Check sheet for the modelled part. Datum: model origin and axes. Units: mm. Face numbers are marked on the shaded views. A direction names the side the tool comes from. Coordinates: 2 decimals unless noted, no trailing zeros. Write each loop counter-clockwise with the first axis right and the second up, starting at its lowest first coordinate (ties: lowest second). Pieces come first, ordered by that corner, then holes. Notation, with made-up numbers: (12, 52) -> (51, 52) arc R6 ccw to (51, 60) -> close; hole circle Ø2 at (89, 63.5). An arc over 180 degrees is marked (long way). Put each result on its own line as item: value.
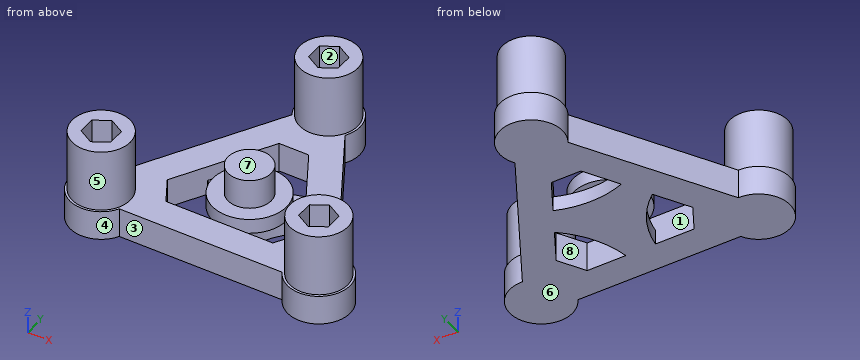
```python
from build123d import *

# Parameters (mm, degrees)
BOSS_EXTRUDE1_DEPTH = 5
BOSS_EXTRUDE2_DEPTH = 5
SKETCH4_R           = 9.75
BOSS_EXTRUDE3_DEPTH = 21
SKETCH5_R           = 12.441578391
BOSS_EXTRUDE4_DEPTH = 5
SKETCH5_3_R         = 7.25
BOSS_EXTRUDE5_DEPTH = 15
CHAMFER1_SIZE       = 10
CUT_EXTRUDE1_DEPTH  = 10


with BuildPart() as part:
    # Sketch2 → Boss-Extrude1 (new body, symmetric)
    with BuildSketch(Plane.XY):
        with BuildLine():
            ThreePointArc((8.946673347, 36.860907204), (0, 52.857), (-8.946673347, 36.860907204))
            Line((-8.946673347, 36.860907204), (-36.395818719, -10.682407204))
            ThreePointArc((-36.395818719, -10.682407204), (-45.775504768, -26.4285), (-27.449145372, -26.1785))
            Line((-27.449145372, -26.1785), (27.449145372, -26.1785))
            ThreePointArc((27.449145372, -26.1785), (45.775504768, -26.4285), (36.395818719, -10.682407204))
            Line((36.395818719, -10.682407204), (8.946673347, 36.860907204))
        make_face()
        Polygon((-28.02198399, -16.1785), (0, 32.357), (28.02198399, -16.1785), align=None, mode=Mode.SUBTRACT)
    extrude(amount=BOSS_EXTRUDE1_DEPTH, both=True)

    # Sketch3 → Boss-Extrude2 (add)
    with BuildSketch(Plane.XY):
        with BuildLine():
            Line((-16.510991995, 3.759122981), (-11.510991995, 12.419377019))
            ThreePointArc((-11.510991995, 12.419377019), (0, 10.282645658), (11.510991995, 12.419377019))
            Line((11.510991995, 12.419377019), (16.510991995, 3.759122981))
            ThreePointArc((16.510991995, 3.759122981), (8.905032358, -5.141322829), (5, -16.1785))
            Line((5, -16.1785), (-5, -16.1785))
            ThreePointArc((-5, -16.1785), (-8.905032358, -5.141322829), (-16.510991995, 3.759122981))
        make_face()
    extrude(amount=-BOSS_EXTRUDE2_DEPTH)

    # Sketch4 → Boss-Extrude3 (add)
    with BuildSketch(Plane.XY.offset(5)):
        with Locations((-36.682238028, -21.1785)):
            Circle(SKETCH4_R)
        with Locations((36.682238028, -21.1785)):
            Circle(SKETCH4_R)
        with Locations((0, 42.357)):
            Circle(SKETCH4_R)
    extrude(amount=BOSS_EXTRUDE3_DEPTH)

    # Sketch5 → Boss-Extrude4 (add)
    with BuildSketch(Plane.XY):
        Circle(SKETCH5_R)
    extrude(amount=BOSS_EXTRUDE4_DEPTH)

    # Sketch5<3> → Boss-Extrude5 (add)
    with BuildSketch(Plane.XY):
        Circle(SKETCH5_3_R)
    extrude(amount=BOSS_EXTRUDE5_DEPTH)

    # Chamfer1
    chamfer1_edges = [part.edges().sort_by_distance(p)[0] for p in [
        (28.02198399, -16.1785, 0),
        (-28.02198399, -16.1785, 0),
        (0, 32.357, 0),
    ]]
    chamfer(chamfer1_edges, length=CHAMFER1_SIZE)

    # Sketch8 → Cut-Extrude1 (cut)
    with BuildSketch(Plane.XY.offset(26)):
        Polygon((-41.682238028, -24.065251346), (-36.682238028, -26.952002692), (-31.682238028, -24.065251346), (-31.682238028, -18.291748654), (-36.682238028, -15.404997308), (-41.682238028, -18.291748654), align=None)
        Polygon((41.682238028, -24.065251346), (41.682238028, -18.291748654), (36.682238028, -15.404997308), (31.682238028, -18.291748654), (31.682238028, -24.065251346), (36.682238028, -26.952002692), align=None)
        Polygon((0, 48.130502692), (-5, 45.243751346), (-5, 39.470248654), (0, 36.583497308), (5, 39.470248654), (5, 45.243751346), align=None)
    extrude(amount=-CUT_EXTRUDE1_DEPTH, mode=Mode.SUBTRACT)


solid = part.part
```
Q1. Cross-section at B-B (z = 20). State how many separate pieces and enclosed holes the cut face has, plus the area to 3 significant figures.
Recorded:
separate pieces: 3
enclosed holes: 3
area: 636 mm2
Q2. Tool access check on the marked faces 5, 6, 7 and 8. Record the directions out of +Z, -Z, +X, -X, +Y, -Y that give a thin tool (end or side, any length) a straight path to the whole face; none if there is none.
Recorded:
face 5: +Z
face 6: -Z, +X, -X, +Y, -Y
face 7: +Z, +X, -X, -Y
face 8: +Z, -Z
Q3. Cross-section at A-A (z = 3.5). Record the cut outline in (x, y).
Recorded:
outline: (-36.4, -10.68) arc R10.5 ccw (long way) to (-27.45, -26.18) -> (27.45, -26.18) arc R10.5 ccw (long way) to (36.4, -10.68) -> (8.95, 36.86) arc R10.5 ccw (long way) to (-8.95, 36.86) -> close; circle Ø24.88 at (0, 0); hole (-23.02, -7.52) -> (-18.02, -16.18) -> (18.02, -16.18) -> (23.02, -7.52) -> (5, 23.7) -> (-5, 23.7) -> close
Q4. Material ranges on line 1 along X through (y, z) = (-19, 19.5); line 2 along X through (y, z) = (44, 23); line 3 along X through (y, z) = (-18.5, 22.5), recorded low to high.
Recorded:
line 1: x = -46.19 to -41.68, -31.68 to -27.18, 27.18 to 31.68, 41.68 to 46.19
line 2: x = -9.61 to -5, 5 to 9.61
line 3: x = -46.06 to -41.68, -31.68 to -27.31, 27.31 to 31.68, 41.68 to 46.06
Q5. Cross-section at D-D (x = 20). Record the cut outline in (y, z).
Recorded:
outline: (-26.18, -5) -> (-12.75, -5) -> (-12.75, 5) -> (-26.18, 5) -> close; (-2.28, -5) -> (17.72, -5) -> (17.72, 5) -> (-2.28, 5) -> close
Q6. Depth check by flat-ended pin: P1, Ø5, axis at x = 35.5, y = -22.5, coming from the +Z side; P2, Ø3, axis at x = -1.5, z = -1.5, coming from the -Y side; P3, Ø20, axis at x = -4, y = 0, coming from the +Z side; P4, Ø10, axis at x = 17.5, z = 15.5, coming from the +Y side. Enter the tip coordinate at first touch or a pass-through.
Recorded:
P1: stops at z = 16
P2: stops at y = -26.18
P3: stops at z = 15
P4: passes through
Q7. Cross-section at C-C (y = -2.5). Record the cut outline in (x, z), plus the area to 3 significant figures.
Recorded:
outline: (-31.67, -5) -> (-20.12, -5) -> (-20.12, 5) -> (-31.67, 5) -> close; (-12.19, 0) -> (-10.61, 0) -> (-10.61, -5) -> (10.61, -5) -> (10.61, 0) -> (12.19, 0) -> (12.19, 5) -> (6.81, 5) -> (6.81, 15) -> (-6.81, 15) -> (-6.81, 5) -> (-12.19, 5) -> close; (20.12, -5) -> (31.67, -5) -> (31.67, 5) -> (20.12, 5) -> close
area: 595 mm2
Q8. Mould release check, pull along Y, two halves, no side actions. Record for the marked faces 1, 2, 3 and 4: released by +Y, released by -Y, zero draft, split by the parting line, or undercut.
Recorded:
face 1: undercut
face 2: undercut
face 3: released by -Y
face 4: split by the parting line
